Geometry check sheet. Reference: the model listing, model coordinates, mm. Round coordinates to 2 decimals unless told otherwise and drop trailing zeros. Loops run counter-clockwise (first coordinate to the right, second up) from the corner with the lowest first, then second, coordinate; pieces in that order, holes last.
```python
from build123d import *

# Parameters (mm, degrees)
SKETCH_1_R          = 1
EXTRUDE_1_DEPTH     = 1.6
SKETCH_2_W          = 1.78
SKETCH_2_H          = 8.1
CUT_EXTRUDE_1_DEPTH = 0.1
CUT_EXTRUDE_START   = 1.6
SKETCH_3_W          = 1.78
SKETCH_3_H          = 8.1
CUT_EXTRUDE_2_DEPTH = 0.1
SKETCH_4_W          = 23
SKETCH_4_H          = 2.54
EXTRUDE_2_DEPTH     = 2
EXTRUDE_START       = 15
SKETCH_5_W          = 0.5
SKETCH_5_H          = 0.5
EXTRUDE_3_DEPTH     = 7


with BuildPart() as part:
    # 草图1 → 凸台-拉伸1 (new body)
    with BuildSketch(Plane.XY):
        with BuildLine():
            Line((-12.5, 0), (-7.62, 0))
            Line((-7.62, 0), (-7.62, -9.41))
            ThreePointArc((-7.62, -9.41), (-7.180660172, -10.470660172), (-6.12, -10.91))
            Line((-6.12, -10.91), (6.12, -10.91))
            ThreePointArc((6.12, -10.91), (7.180660172, -10.470660172), (7.62, -9.41))
            Line((7.62, -9.41), (7.62, 0))
            Line((7.62, 0), (12.5, 0))
            Line((12.5, 0), (12.5, 15))
            Line((12.5, 15), (-12.5, 15))
            Line((-12.5, 15), (-12.5, 0))
        make_face()
        with Locations((-10, 8)):
            Circle(SKETCH_1_R, mode=Mode.SUBTRACT)
        with Locations((10, 8)):
            Circle(SKETCH_1_R, mode=Mode.SUBTRACT)
    extrude(amount=EXTRUDE_1_DEPTH)

    # 草图2 → 切除-拉伸1 (cut)
    with BuildSketch(Plane.XY):
        with Locations((0, -6.36)):
            Rectangle(SKETCH_2_W, SKETCH_2_H)
        with Locations((2.54, -6.36)):
            Rectangle(SKETCH_2_W, SKETCH_2_H)
        with Locations((5.08, -6.36)):
            Rectangle(SKETCH_2_W, SKETCH_2_H)
        with Locations((-2.54, -6.36)):
            Rectangle(SKETCH_2_W, SKETCH_2_H)
        with Locations((-5.08, -6.36)):
            Rectangle(SKETCH_2_W, SKETCH_2_H)
    extrude(amount=CUT_EXTRUDE_1_DEPTH, mode=Mode.SUBTRACT)

    # 草图3 → 切除-拉伸2 (cut)
    with BuildSketch(Plane.XY.offset(CUT_EXTRUDE_START)):
        with Locations((2.54, -6.36)):
            Rectangle(SKETCH_3_W, SKETCH_3_H)
        with Locations((0, -6.36)):
            Rectangle(SKETCH_3_W, SKETCH_3_H)
        with Locations((-5.08, -6.36)):
            Rectangle(SKETCH_3_W, SKETCH_3_H)
        with Locations((-2.54, -6.36)):
            Rectangle(SKETCH_3_W, SKETCH_3_H)
        with Locations((5.08, -6.36)):
            Rectangle(SKETCH_3_W, SKETCH_3_H)
    extrude(amount=-CUT_EXTRUDE_2_DEPTH, mode=Mode.SUBTRACT)

    # 草图4 → 凸台-拉伸2 (add)
    with BuildSketch(Plane.XY):
        with Locations((0, 13.73)):
            Rectangle(SKETCH_4_W, SKETCH_4_H)
    extrude(amount=-EXTRUDE_2_DEPTH)

    # 草图5 → 凸台-拉伸3 (add)
    with BuildSketch(Plane(origin=(0, 0, 0), x_dir=(1, 0, 0), z_dir=(0, 1, 0)).offset(EXTRUDE_START)):
        with Locations((2.54, 1)):
            Rectangle(SKETCH_5_W, SKETCH_5_H)
        with Locations((0, 1)):
            Rectangle(SKETCH_5_W, SKETCH_5_H)
        with Locations((5.08, 1)):
            Rectangle(SKETCH_5_W, SKETCH_5_H)
        with Locations((7.62, 1)):
            Rectangle(SKETCH_5_W, SKETCH_5_H)
        with Locations((10.16, 1)):
            Rectangle(SKETCH_5_W, SKETCH_5_H)
        with Locations((-2.54, 1)):
            Rectangle(SKETCH_5_W, SKETCH_5_H)
        with Locations((-5.08, 1)):
            Rectangle(SKETCH_5_W, SKETCH_5_H)
        with Locations((-7.62, 1)):
            Rectangle(SKETCH_5_W, SKETCH_5_H)
        with Locations((-10.16, 1)):
            Rectangle(SKETCH_5_W, SKETCH_5_H)
    extrude(amount=EXTRUDE_3_DEPTH)


solid = part.part
```
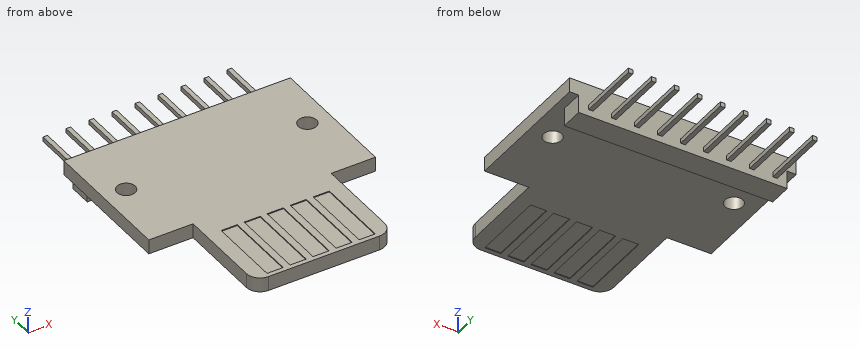
1) Sectioned sample at A-A, the plane y = 8. Record the cut outline in (x, z), then the cut area to 3 significant figures.
Report:
outline: (-12.5, 0) - (-11, 0) - (-11, 1.6) - (-12.5, 1.6) - close; (-9, 0) - (9, 0) - (9, 1.6) - (-9, 1.6) - close; (11, 0) - (12.5, 0) - (12.5, 1.6) - (11, 1.6) - close
area: 33.6 mm2
2) Gauge pin test, flat ends, axial feed: pin 1 (0.5 mm diameter, centred on x = -2.5, y = -5, fed in from -Z); pin 2 (2.5 mm diameter, centred on x = 10, y = 8, fed in from -Z); pin 3 (1 mm diameter, centred on x = 7.5, z = 1, fed in from -Y). Record the tip position at first contact, or that the pin passes through.
Report:
pin 1: stops at z = 0.1
pin 2: stops at z = 0
pin 3: stops at y = -10.62
3) Sectioned sample at C-C, the plane z = -0.4. Record the cut outline in (x, y), then the cut area to 3 significant figures.
Report:
outline: (-11.5, 12.46) - (11.5, 12.46) - (11.5, 15) - (-11.5, 15) - close
area: 58.4 mm2
4) Sectioned sample at D-D, the plane y = 16. State how many separate pieces and enclosed holes the cut face has, then the cut area to 3 significant figures.
Report:
separate pieces: 9
enclosed holes: 0
area: 2.25 mm2
5) Scan lines: line 1 along Y through (x, z) = (10, 1); line 2 along Y through (x, z) = (2.5, -0.5); line 3 along Y through (x, z) = (5.25, 1.05). Record each from-to range of solid material in increasing order.
Report:
line 1: y = 0 to 7, 9 to 15
line 2: y = 12.46 to 15
line 3: y = -10.91 to 15
6) Sectioned sample at B-B, the plane x = 1.25. Record the cut outline in (y, z).
Report:
outline: (-10.91, 0) - (12.46, 0) - (12.46, -2) - (15, -2) - (15, 1.6) - (-10.91, 1.6) - close
